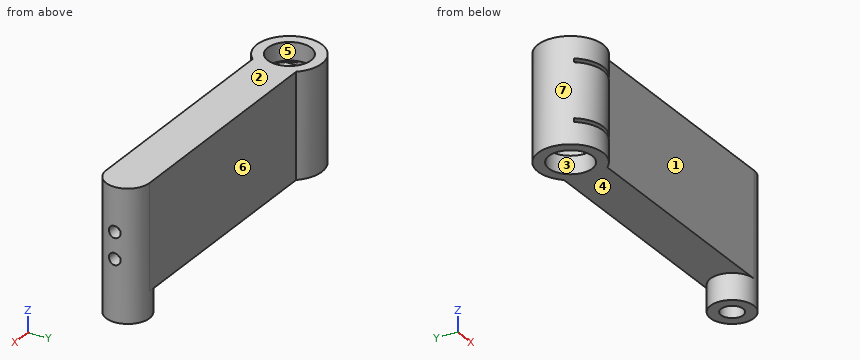
Autodesk Fusion 360 part; units mm, degrees
sketch "スケッチ1" plane through (0, 0, 0) normal (0, 0, 1) x (1, 0, 0)
  line L0 (0, 0) -> (60, 0)
  line L1 (60, 0) -> (60, 10)
  line L2 (60, 10) -> (0, 10)
  line L3 (0, 10) -> (0, 0)
  circle A0 centre (0, 5) radius 7.5
  dimension "d1" = 15
sketch "スケッチ2" plane through (0, 0, 0) normal (0, 0, 1) x (1, 0, 0)
sketch "スケッチ3" plane through (0, 0, 0) normal (0, 0, 1) x (1, 0, 0)
sketch "スケッチ4" plane through (0, 0, 0) normal (0, 0, 1) x (1, 0, 0)
  circle A0 centre (60, 5) radius 5
extrude "押し出し1" add sketch "スケッチ4" sketch "スケッチ1" along normal blind 24 of sketch 2
sketch "スケッチ5" plane through (0, 0, 0) normal (0, 0, -1) x (1, 0, 0)
  arc A0 (60, -10) -> (60, 0) centre (60, -5) ccw
  line L0 (60, 0) -> (5.5902, 0)
  arc A1 (5.5902, 0) -> (5.5902, -10) centre (0, -5) ccw
  line L1 (5.5902, -10) -> (60, -10)
  circle A2 centre (60, -5) radius 5
extrude "押し出し2" add sketch "スケッチ5" along normal blind 6 contours A0 A2
sketch "スケッチ6" plane through (0, 0, 0) normal (0, 0, -1) x (1, 0, 0)
  arc A0 (60, 0) -> (60, -10) centre (60, -5) ccw
  line L0 (60, 0) -> (5.5902, 0)
  arc A1 (5.5902, 0) -> (5.5902, -10) centre (0, -5) ccw
  line L1 (5.5902, -10) -> (60, -10)
  circle A2 centre (0, -5) radius 5
  dimension "d6" = 10
extrude "押し出し3" cut sketch "スケッチ6" against normal blind 4.1 contours A2
sketch "スケッチ7" plane through (0, 0, 24) normal (0, 0, 1) x (-1, 0, 0)
  arc A0 (-60, 0) -> (-60, -10) centre (-60, -5) ccw
  line L0 (-60, -10) -> (-5.5902, -10)
  arc A1 (-5.5902, -10) -> (-5.5902, 0) centre (0, -5) ccw
  line L1 (-5.5902, 0) -> (-60, 0)
  circle A2 centre (0, -5) radius 5
  dimension "d9" = 10
extrude "押し出し4" cut sketch "スケッチ7" against normal blind 4.1 contours A2
sketch "スケッチ8" plane through (0, 0, 0) normal (0, 1, 0) x (1, 0, 0)
sketch "スケッチ9" plane through (0, 0, 0) normal (0, 1, 0) x (1, 0, 0)
sketch "スケッチ10" plane through (0, 0, 4.1) normal (0, 0, -1) x (1, 0, 0)
  circle A0 centre (0, -5) radius 5
  circle A1 centre (0, -5) radius 6
  dimension "d12" = 12
extrude "押し出し5" cut sketch "スケッチ10" against normal blind 0.85 contours A0 | A1
extrude "押し出し6" cut 1 faces at (-0.8908, 6.4538, 4.95) along direction (0, 0, 1) blind 0.85
sketch "スケッチ11" plane through (0, 0, 19.9) normal (0, 0, 1) x (-1, 0, 0)
  circle A0 centre (0, -5) radius 5
  circle A1 centre (0, -5) radius 6
  dimension "d17" = 12
extrude "押し出し7" cut sketch "スケッチ11" against normal blind 0.85 contours A0 | A1
extrude "押し出し8" cut 1 faces at (1.5116, 5.0736, 19.05) along direction (0, 0, -1) blind 0.85
sketch "スケッチ19" plane through (0, 0, 18.2) normal (0, 0, 1) x (-1, 0, 0)
  circle A0 centre (0, -5) radius 6
  line L0 (-6, -5) -> (6, -5)
  line L1 (6, -5) -> (6, -10)
  line L2 (6, -10) -> (-6, -10)
  line L3 (-6, -10) -> (-6, -5)
sketch "スケッチ20" plane through (0, 0, 0) normal (0, 1, 0) x (1, 0, 0)
  line L0 (6, -18.2) -> (-6, -18.2)
  line L1 (-6, -18.2) -> (-6, -19.05)
  line L2 (-6, -19.05) -> (6, -19.05)
  line L3 (6, -19.05) -> (6, -18.2)
  dimension "d27" = 0.85
extrude "押し出し9" cut sketch "スケッチ20" against normal blind 2.5
sketch "スケッチ21" plane through (0, 0, 0) normal (0, -1, 0) x (1, 0, 0)
  line L0 (5.5902, 18.2) -> (5.5902, 0)
  line L1 (5.5902, 0) -> (60, 0)
  line L2 (60, 0) -> (60, 24)
  line L3 (60, 24) -> (5.5902, 24)
  line L4 (5.5902, 24) -> (5.5902, 19.05)
  line L5 (5.5902, 19.05) -> (3.3166, 19.05)
  line L6 (3.3166, 19.05) -> (3.3166, 18.2)
  line L7 (3.3166, 18.2) -> (5.5902, 18.2)
  line L8 (6, 18.2) -> (3.3166, 18.2)
  line L9 (3.3166, 18.2) -> (3.3166, 19.05)
  line L10 (3.3166, 19.05) -> (6, 19.05)
  line L11 (6, 19.05) -> (6, 18.2)
  line L12 (-6, 18.2) -> (-3.308, 18.2)
  line L13 (-3.308, 18.2) -> (-3.308, 19.05)
  line L14 (-3.308, 19.05) -> (-6, 19.05)
  line L15 (-6, 19.05) -> (-6, 18.2)
extrude "押し出し10" cut sketch "スケッチ21" against normal blind 5 contours L5 L6 L7 L8 L9 L10 L11 | L12 L13 L14 L15
sketch "スケッチ22" plane through (0, 0, 5.8) normal (0, 0, -1) x (1, 0, 0)
  circle A0 centre (0, -5) radius 6
  line L0 (6, -5) -> (-6, -5)
  line L1 (-6, -5) -> (-6, 0)
  line L2 (-6, 0) -> (6, 0)
  line L3 (6, 0) -> (6, -5)
sketch "スケッチ23" plane through (0, 0, 0) normal (0, 1, 0) x (1, 0, 0)
  line L0 (6, -5.8) -> (-6, -5.8)
  line L1 (-6, -5.8) -> (-6, -4.95)
  line L2 (-6, -4.95) -> (6, -4.95)
  line L3 (6, -4.95) -> (6, -5.8)
  dimension "d32" = 0.85
extrude "押し出し11" cut sketch "スケッチ23" against normal blind 2.5
sketch "スケッチ24" plane through (0, 0, 0) normal (0, -1, 0) x (1, 0, 0)
  line L0 (5.5902, 4.95) -> (5.5902, 0)
  line L1 (5.5902, 0) -> (60, 0)
  line L2 (60, 0) -> (60, 24)
  line L3 (60, 24) -> (5.5902, 24)
  line L4 (5.5902, 24) -> (5.5902, 19.05)
  line L5 (5.5902, 19.05) -> (6, 19.05)
  line L6 (6, 19.05) -> (6, 18.2)
  line L7 (6, 18.2) -> (5.5902, 18.2)
  line L8 (5.5902, 18.2) -> (5.5902, 5.8)
  line L9 (5.5902, 5.8) -> (3.3166, 5.8)
  line L10 (3.3166, 5.8) -> (3.3166, 4.95)
  line L11 (3.3166, 4.95) -> (5.5902, 4.95)
  line L12 (6, 5.8) -> (3.3166, 5.8)
  line L13 (3.3166, 5.8) -> (3.3166, 4.95)
  line L14 (3.3166, 4.95) -> (6, 4.95)
  line L15 (6, 4.95) -> (6, 5.8)
  line L16 (-6, 5.8) -> (-3.3133, 5.8)
  line L17 (-3.3133, 5.8) -> (-3.3133, 4.95)
  line L18 (-3.3133, 4.95) -> (-6, 4.95)
  line L19 (-6, 4.95) -> (-6, 5.8)
extrude "押し出し12" cut sketch "スケッチ24" against normal blind 5 contours L9 L10 L11 L12 L13 L14 L15 | L16 L17 L18 L19
sketch "スケッチ25" plane through (0, 0, -6) normal (0, 0, -1) x (1, 0, 0)
  circle A0 centre (60, -5) radius 5
  circle A1 centre (60, -5) radius 2.55
  dimension "d37" = 5.1
extrude "押し出し13" cut sketch "スケッチ25" against normal blind 25.4 contours A1
sketch "スケッチ26" plane through (0, 0, 19.4) normal (0, 0, -1) x (1, 0, 0)
  circle A0 centre (60, -5) radius 2.55
  line L0 (62.55, -5) -> (61.95, -5)
  line L1 (61.95, -5) -> (61.95, -6.6432)
  line L2 (61.95, -5) -> (61.95, -3.3568)
  dimension "d40" = 0.6
extrude "押し出し14" add sketch "スケッチ26" along normal blind 21.4 contours A0 L0 L2 | A0 L0 L1
sketch "スケッチ27" plane through (61.95, 0, 0) normal (-1, 0, 0) x (0, -1, 0)
  line L0 (-3.3568, 19.4) -> (-6.6432, 19.4)
  line L1 (-6.6432, 19.4) -> (-6.6432, -2)
  line L2 (-6.6432, -2) -> (-3.3568, -2)
  line L3 (-3.3568, -2) -> (-3.3568, 19.4)
  circle A0 centre (-5, 14) radius 1.35
  circle A1 centre (-5, 8) radius 1.35
  dimension "d43" = 2.7
  dimension "d44" = 2.7
extrude "押し出し15" cut sketch "スケッチ27" against normal blind 3.5 contours A0 | A1
sketch "スケッチ28" plane through (0, 0, 5.8) normal (0, 0, -1) x (1, 0, 0)
  circle A0 centre (0, -5) radius 2.75
  dimension "d47" = 5.5
extrude "押し出し16" cut sketch "スケッチ28" against normal blind 15
Here's how the part is built. I have some questions about the finished solid (model axes, mm). Face numbers are marked on the shaded views. A direction names the side the tool comes from. Coordinates: 2 decimals unless noted, no trailing zeros. Write each loop counter-clockwise with the first axis right and the second up, starting at its lowest first coordinate (ties: lowest second). Pieces come first, ordered by that corner, then holes. Notation, with made-up numbers: (-10, 62) - (48, 62) arc R17 ccw to (48, 68) - close; hole circle Ø1 at (19.5, 40). An arc over 180 degrees is marked (long way). Use one line per item in the form item = value.
1) Suppose I cut it at A-A, the plane x = 0. Write out the boundary of the cut face in (y, z), plus the area to 3 significant figures.
Solved:
outline = (-2.5, 0) - (0, 0) - (0, 4.1) - (-1, 4.1) - (-1, 4.95) - (-2.5, 4.95) - close; (-2.5, 5.8) - (2.25, 5.8) - (2.25, 18.2) - (-2.5, 18.2) - close; (-2.5, 19.05) - (-1, 19.05) - (-1, 19.9) - (0, 19.9) - (0, 24) - (-2.5, 24) - close; (7.75, 5.8) - (11, 5.8) - (11, 4.1) - (10, 4.1) - (10, 0) - (12.5, 0) - (12.5, 24) - (10, 24) - (10, 19.9) - (11, 19.9) - (11, 18.2) - (7.75, 18.2) - close
area = 166 mm2
2) On a 3-axis mill with a long thin cutter (end or side, diameter ignored), from which of +Z, -Z, +X, -X, +Y, -Y can I reach the whole of each face in a straight line? I mean the marked faces 1, 2 and 3. Say none if no direction works.
Solved:
face_1 = +Z, -Z, +X, -Y
face_2 = +Z, +X, -X, +Y, -Y
face_3 = -Z
3) Thinking about a two-plate mould opening in Y: for the marked faces 4, 5, 6 and 7, which applies, released by +Y, released by -Y, zero draft, split by the parting line, or undercut?
Solved:
face_4 = zero draft
face_5 = undercut
face_6 = released by +Y
face_7 = split by the parting line
4) Suppose I cut it at B-B, the plane z = 21. Write out the boundary of the cut face in (x, y), plus the area to 3 significant figures.
Solved:
outline = (5.59, 0) - (60, 0) arc R5 ccw to (60, 10) - (5.59, 10) arc R7.5 ccw (long way) to start; hole circle Ø10 at (0, 5)
area = 668 mm2
5) Suppose I cut it at C-C, the plane z = 2. Write out the boundary of the cut face in (x, y), plus the area to 3 significant figures.
Solved:
outline = (5.59, 0) - (60, 0) arc R5 ccw to (60, 10) - (5.59, 10) arc R7.5 ccw (long way) to start; hole circle Ø10 at (0, 5); hole (61.95, 3.36) - (61.95, 6.64) arc R2.55 ccw (long way) to start
area = 649 mm2
6) I need wall thicknesses on line 1 (Z direction, x = -0.5, y = -1.25); line 2 (X direction, y = 5, z = 12.5); line 3 (X direction, y = 5, z = 4.65). Which ranges of each line are inside material? Lowest first, please.
Solved:
line_1 = 0 to 4.95, 5.8 to 18.2, 19.05 to 24
line_2 = -7.5 to -2.75, 2.75 to 57.45, 61.95 to 65
line_3 = -7.5 to -6, 6 to 57.45, 61.95 to 65
7) Suppose I cut it at D-D, the plane y = 8.75. Write out the boundary of the cut face in (x, z).
Solved:
outline = (-6.5, 0) - (-3.31, 0) - (-3.31, 4.1) - (-4.68, 4.1) - (-4.68, 5.8) - (4.68, 5.8) - (4.68, 4.1) - (3.31, 4.1) - (3.31, 0) - (56.69, 0) - (56.69, -6) - (63.31, -6) - (63.31, 24) - (3.31, 24) - (3.31, 19.9) - (4.68, 19.9) - (4.68, 18.2) - (-4.68, 18.2) - (-4.68, 19.9) - (-3.31, 19.9) - (-3.31, 24) - (-6.5, 24) - close
8) I'm going to push flat-ended pins straight in: P1, Ø1, axis at x = 29.5, y = 0.5, coming from the -Z side; P2, Ø2, axis at x = 24, z = 8.5, coming from the -Y side; P3, Ø0.9, axis at y = 2.5, z = 19, coming from the +X side; P4, Ø3, axis at x = 19.5, z = -2.5, coming from the -Y side. Where does each tip first touch, or does it pass through?
Solved:
P1 = 0
P2 = 0
P3 = 64.56
P4 = through
